Input: part model. Units: mm. Frame: model coordinates. A direction names the side the tool comes from. Round coordinates to 2 decimals unless told otherwise and drop trailing zeros. Loops run counter-clockwise (first coordinate to the right, second up) from the corner with the lowest first, then second, coordinate; pieces in that order, holes last. Notation, with made-up numbers: (42.5, 5) -> (77.5, 5) arc R5 cw to (77.5, 12) -> close; hole circle Ø9 at (51, 65). An arc over 180 degrees is marked (long way). One line per question, with ' | ' between items. Start each with the question number.
Q1. Cut plane A-A on z = 145. Return loops of the section in (x, y), and give its area (3 significant figures).
Q2. Access query for faces 1 (the face through (-7.042, -18.14, 149.694)), 2 (the face through (-147.27, -13.57, 48.59)). Directions: +Z, -Z, +X, -X, +Y, -Y. A direction counts if a zero-diameter tool reaches every point of the face in a straight line with its end or side. Return the directions, or none.
Q3. Cut plane B-B on y = -13.5. State how many separate pieces and enclosed holes the cut face has, and give its area (3 significant figures).
Q4. Cut plane C-C on x = -113.5. Return loops of the section in (y, z), and give its area (3 significant figures).
Q5. Cut plane D-D on z = 82. Return loops of the section in (x, y), and give its area (3 significant figures).
Q6. Mould query, pull axis X, two halves, no side actions, for faces 3 (the face through (-37.878, -13.64, 119.276)), 4 (the face through (-67, -3.5, 95)), 5 (the face through (-66.65, -13.36, 87.51)). Classes: pulls with the +X half, pulls with the -X half, needs draft (parallel to the pull), parting line crosses it, or undercut.
Q7. Contact query for flat-ended pins moving along their axis: P1, Ø1.5, axis at y = -17, z = 120, coming from the -X side; P2, Ø1.6, axis at x = -5.5, y = -14, coming from the -Z side; P3, Ø5, axis at y = -21, z = 91, coming from the -X side; P4, Ø4.5, axis at x = -39.4, z = 121.26, coming from the -Y side. Output: stop coordinate, or through.
Q8. Material intervals for L1, parallel to Z at x = -1.15, y = -13.5; L2, parallel to Y at x = -2.4, z = 145; L3, parallel to X at y = -17.75, z = 145.5, sorted ascending.
Autodesk Inventor part; units mm, degrees
ref_plane "YZ Plane" through (0, 0, 0) normal (1, 0, 0) x (0, 1, 0)
ref_plane "XZ Plane" through (0, 0, 0) normal (0, 1, 0) x (-1, 0, 0)
ref_plane "XY Plane" through (0, 0, 0) normal (0, 0, 1) x (1, 0, 0)
sketch "Sketch1" plane through (0, 0, 0) normal (0, 1, 0) x (-1, 0, 0)
  circle A0 centre (0, 0) radius 135
  circle A1 centre (0, 0) radius 110
  dimension "d0" = 270
  dimension "d1" = 220
extrude "Extrusion1" add sketch "Sketch1" along normal mid plane 47
sketch "Sketch2" plane through (0, 0, 0) normal (0, 0, 1) x (1, 0, 0)
  circle A0 centre (0, -20.5) radius 18
  line L0 (-135, -23.5) -> (135, -23.5)
  dimension "d4" = 36
  dimension "d38" = 3
extrude "Extrusion2" cut sketch "Sketch2" against normal through all
sketch "Sketch3" plane through (0, 23.5, 0) normal (0, 1, 0) x (1, 0, 0)
  circle A0 centre (0, 0) radius 127.5
  circle A1 centre (-127.5, 0) radius 2
  circle A2 centre (-103.1497, -74.9426) radius 2
  circle A3 centre (-39.3997, -121.2597) radius 2
  circle A4 centre (39.3997, -121.2597) radius 2
  circle A5 centre (103.1497, -74.9426) radius 2
  circle A6 centre (127.5, 0) radius 2
  circle A7 centre (103.1497, 74.9426) radius 2
  circle A8 centre (39.3997, 121.2597) radius 2
  circle A9 centre (-39.3997, 121.2597) radius 2
  circle A10 centre (-103.1497, 74.9426) radius 2
  dimension "d7" = 255
  dimension "d8" = 4
  dimension "d11" = 360
hole "Hole1" at (39.3997, 23.5, 121.2597) at (-39.3997, 23.5, 121.2597) at (-103.1497, 23.5, 74.9426) at (-127.5, 23.5, 0) at (-103.1497, 23.5, -74.9426) at (-39.3997, 23.5, -121.2597) at (39.3997, 23.5, -121.2597) at (103.1497, 23.5, -74.9426) at (127.5, 23.5, 0) at (103.1497, 23.5, 74.9426) direction (0, -1, 0) diameter 5 end through all
sketch "Sketch4" plane through (0, 23.5, 0) normal (0, 1, 0) x (1, 0, 0)
  circle A0 centre (0, 0) radius 140
extrude "Extrusion3" cut sketch "Sketch4" against normal blind 27
sketch "Sketch7" plane through (0, -3.5, 0) normal (0, 1, 0) x (1, 0, 0)
  line L0 (0, 0) -> (70, 0)
  line L1 (80, -100) -> (60, -100)
  line L2 (60, -100) -> (60, 100)
  line L3 (60, 100) -> (80, 100)
  line L4 (80, 100) -> (80, -100)
  line L5 (80, -100) -> (60, 100) construction
  line L6 (60, -100) -> (80, 100) construction
  dimension "d39" = 70
  dimension "d40" = 20
  dimension "d41" = 200
extrude "Extrusion7" cut sketch "Sketch7" against normal blind 15
sketch "Sketch8" plane through (0, -3.5, 0) normal (0, 1, 0) x (1, 0, 0)
  line L0 (-129.4827, -38.1999) -> (129.4827, 38.1999)
  line L1 (0, 134.8703) -> (0, -135)
  arc A0 (-5.9161, 134.8703) -> (5.9161, 134.8703) centre (0, 0) ccw
  arc A1 (5.9161, 134.8703) -> (-5.9161, 134.8703) centre (0, 0) ccw
  point P0 (5.9161, 134.8703)
  point P1 (0, 0)
extrude "Extrusion8" cut sketch "Sketch8" against normal through all contours A0 A1 L0 | L0 A0 L1 picked at (87.5063, 20.3809)
sketch "Sketch9" plane through (-129.4827, -23.5, 38.1999) normal (-0.2829619, 0, -0.9591312) x (-0.9591312, 0, 0.2829619)
  line L0 (-96.8001, 0) -> (0, 0)
  line L1 (-2.5, 0) -> (15, 0)
  line L2 (20, 5) -> (20, 15)
  line L3 (15, 20) -> (-2.5, 20)
  line L4 (-2.5, 20) -> (-2.5, 0)
  line L5 (0, 20) -> (0, 0)
  arc A0 (20, 15) -> (15, 20) centre (15, 15) ccw
  arc A1 (15, 0) -> (20, 5) centre (15, 5) ccw
  point P0 (-135, 23.5)
  point P1 (20, 20)
  point P2 (20, 0)
  dimension "d46" = 22.5
  dimension "d47" = 20
  dimension "d48" = 20
  dimension "d49" = 5
extrude "Extrusion9" add sketch "Sketch9" against normal blind 10
fillet "Fillet1" radius 2.5 1 edges at (-126.2974, -13.5, 47.6862)
sketch "Sketch10" plane through (-126.6531, -23.5, 47.7912) normal (0.2829619, 0, 0.9591312) x (0.9591312, 0, -0.2829619)
  line L0 (-20, 15) -> (-20, 5)
  line L1 (-1.9306, 20) -> (-15, 20)
  point P0 (135, 23.5)
  point P1 (-10, 10)
  dimension "d53" = 10
  dimension "d54" = 10
hole "Hole2" at (-136.2444, -13.5, 50.6208) direction (-0.2829619, 0, -0.9591312) diameter 8.2 end through all counterbore diameter 13.2 counterbore depth 6
sketch "Sketch11" plane through (0, -3.5, 135) normal (1, 0, 0) x (0, 0, -1)
  line L0 (2.5, 0) -> (-15, 0)
  line L1 (-20, -5) -> (-20, -15)
  line L2 (-15, -20) -> (2.5, -20)
  line L3 (2.5, -20) -> (2.5, 0)
  line L4 (0, -20) -> (0, 0)
  arc A0 (-15, 0) -> (-20, -5) centre (-15, -5) ccw
  arc A1 (-20, -15) -> (-15, -20) centre (-15, -15) ccw
  point P0 (135, 3.5)
  point P1 (-20, -20)
  point P2 (-20, 0)
  dimension "d62" = 22.5
  dimension "d63" = 20
  dimension "d64" = 20
  dimension "d65" = 5
extrude "Extrusion10" add sketch "Sketch11" against normal blind 10
fillet "Fillet2" radius 2.5 1 edges at (-10, -13.5, 134.6291)
sketch "Sketch12" plane through (-10, -3.5, 135) normal (-1, 0, 0) x (0, 0, 1)
  line L0 (16.6, -12.7338) -> (12.7338, -16.6)
  line L1 (12.7338, -16.6) -> (7.2662, -16.6)
  line L2 (7.2662, -16.6) -> (3.4, -12.7338)
  line L3 (3.4, -12.7338) -> (3.4, -7.2662)
  line L4 (3.4, -7.2662) -> (7.2662, -3.4)
  line L5 (7.2662, -3.4) -> (12.7338, -3.4)
  line L6 (12.7338, -3.4) -> (16.6, -7.2662)
  line L7 (16.6, -7.2662) -> (16.6, -12.7338)
  line L8 (1.9306, -20) -> (15, -20)
  line L9 (20, -15) -> (20, -5)
  point P0 (-135, 3.5)
  point P1 (10, -10)
  dimension "d69" = 10
  dimension "d70" = 10
  dimension "d71" = 13.2
extrude "Extrusion11" cut sketch "Sketch12" against normal blind 6
sketch "Sketch13" plane through (-4, -3.5, 135) normal (-1, 0, 0) x (0, 0, 1)
  line L0 (20, -15) -> (20, -5)
  point P0 (-135, 3.5)
  point P1 (10, -10)
  dimension "d74" = 10
hole "Hole3" at (-4, -13.5, 145) direction (1, 0, 0) diameter 8.2 end through all
properties part number "Cylinder Spacer Bottom_Q4"
Results:
1) outline: (-10, -23.5) -> (0, -23.5) -> (0, -17.6) -> (-4, -17.6) -> (-4, -20.1) -> (-10, -20.1) -> close; (-10, -6.9) -> (-4, -6.9) -> (-4, -9.4) -> (0, -9.4) -> (0, -3.5) -> (-10, -3.5) -> close | area: 88.0 mm^2
2) face 1: -X | face 2: +Z, -X, +Y, -Y
3) separate pieces: 3 | enclosed holes: 2 | area: 4,070 mm^2
4) outline: (-23.5, 33.48) -> (-3.5, 33.48) -> (-3.5, 73.09) -> (-23.5, 73.09) -> close | area: 792 mm^2
5) outline: (-107.24, -23.5) -> (-73.32, -23.5) -> (-73.32, -3.5) -> (-107.24, -3.5) -> close | area: 678 mm^2
6) face 3: undercut | face 4: needs draft | face 5: pulls with the +X half
7) P1: x = -63.28 | P2: z = 109.82 | P3: x = -101.94 | P4: through
8) L1: 109.99 to 140.9, 149.1 to 155 | L2: -23.5 to -17.6, -9.4 to -3.5 | L3: -4 to 0
